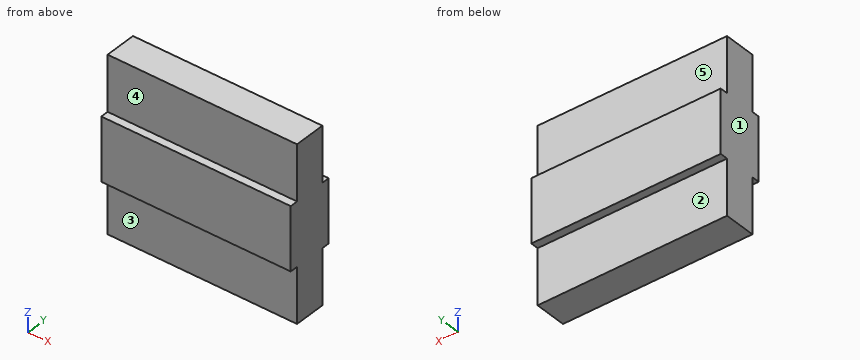
```python
from build123d import *

# Parameters (mm, degrees)
F0_W     = 304.8
F0_H     = 101.6
F1_DEPTH = 38.1
F0_H_2   = 88.9
F2_DEPTH = 25.4


with BuildPart() as f1:
    # F0 (on Front) → F1 (new body, symmetric)
    with BuildSketch(Plane.XZ):
        Rectangle(F0_W, F0_H)
    extrude(amount=F1_DEPTH, both=True)

    # F0 (on Front) → F2 (join, symmetric)
    with BuildSketch(Plane.XZ):
        with Locations((0, 95.25)):
            Rectangle(F0_W, F0_H_2)
        with Locations((0, -95.25)):
            Rectangle(F0_W, F0_H_2)
    extrude(amount=F2_DEPTH, both=True)


solid = f1.part
```
Geometry: final body of the model. Coordinates: model frame, mm. Face numbers are marked on the shaded views. A direction names the side the tool comes from. Coordinates: 2 decimals unless noted, no trailing zeros. Loops run counter-clockwise (first coordinate to the right, second up) from the corner with the lowest first, then second, coordinate; pieces in that order, holes last. Notation, with made-up numbers: (-34.75, 81.5) -> (7.25, 81.5) arc R16 ccw to (7.25, 87.5) -> close; hole circle Ø6 at (46, 11). An arc over 180 degrees is marked (long way). Use a Markdown table: item, result. Add a question column.
(1) Section query B-B, the plane z = -120. Return loops of the section in (x, y), plus the area to 3 significant figures.
(2) Section query A-A, the plane x = -98.5. Return loops of the section in (y, z).
(3) Pin query (flat end, axial travel): pin 1 Ø4 at (x, y) = (68, 30.5) entering from +Z; pin 2 Ø6.5 at (x, y) = (30.5, -31.5) entering from -Z. Return the tip coordinate at first contact, or that it passes through.
(4) Line query: line 1 along Y through (x, z) = (-100.5, 83); line 2 along Z through (x, y) = (54, -30). Output: solid intervals per line, ascending.
(5) Access query for the marked faces 1, 2, 3, 4 and 5. Directions: +Z, -Z, +X, -X, +Y, -Y. A direction counts if a zero-diameter tool reaches every point of the face in a straight line with its end or side. Return the directions, or none.
Answer:
| question | item | result |
|---|---|---|
| 1 | outline | (-152.4, -25.4) -> (152.4, -25.4) -> (152.4, 25.4) -> (-152.4, 25.4) -> close |
| 1 | area | 15,500 mm^2 |
| 2 | outline | (-38.1, -50.8) -> (-25.4, -50.8) -> (-25.4, -139.7) -> (25.4, -139.7) -> (25.4, -50.8) -> (38.1, -50.8) -> (38.1, 50.8) -> (25.4, 50.8) -> (25.4, 139.7) -> (-25.4, 139.7) -> (-25.4, 50.8) -> (-38.1, 50.8) -> close |
| 3 | pin 1 | stops at z = 50.8 |
| 3 | pin 2 | stops at z = -50.8 |
| 4 | line 1 | y = -25.4 to 25.4 |
| 4 | line 2 | z = -50.8 to 50.8 |
| 5 | face 1 | +Z, -Z, -X, +Y, -Y |
| 5 | face 2 | -Z, +X, -X, +Y |
| 5 | face 3 | -Z, +X, -X, -Y |
| 5 | face 4 | +Z, +X, -X, -Y |
| 5 | face 5 | +Z, +X, -X, +Y |
